Design review of the part built by this model. Coordinates are the model's own, in mm. A direction names the side the tool comes from. Coordinates: 2 decimals unless noted, no trailing zeros. Write each loop counter-clockwise with the first axis right and the second up, starting at its lowest first coordinate (ties: lowest second). Pieces come first, ordered by that corner, then holes. Notation, with made-up numbers: (1, -29.5) -> (56, -29.5) arc R34 cw to (56, 9.5) -> close; hole circle Ø5 at (41.5, 63.25). An arc over 180 degrees is marked (long way). Write item = value, one per line. Start each with the question number.
```python
from build123d import *

# Parameters (mm, degrees)
ESBO_O1_R                = 12.5
ESBO_O1_R_2              = 1.5
ESBO_O1_R_3              = 2.5
RESSALTO_EXTRUS_O2_DEPTH = 6
FILETE1_R                = 10
ESBO_O2_R                = 1.5
ESBO_O2_R_2              = 3
ESBO_O2_R_3              = 3.05
CORTE_EXTRUS_O1_DEPTH    = 238.194013415
ESBO_O3_R                = 3
CORTE_EXTRUS_O2_DEPTH    = 238.194013415


with BuildPart() as part:
    # Esboço1 → Ressalto-extrusão2 (new body)
    with BuildSketch(Plane.XY):
        Polygon((0, 0), (0, 215), (50, 215), (100, 0), align=None)
        with Locations((25, 195)):
            Circle(ESBO_O1_R, mode=Mode.SUBTRACT)
        with Locations((25, 211)):
            Circle(ESBO_O1_R_2, mode=Mode.SUBTRACT)
        with Locations((38.856406461, 203)):
            Circle(ESBO_O1_R_2, mode=Mode.SUBTRACT)
        with Locations((38.856406461, 187)):
            Circle(ESBO_O1_R_2, mode=Mode.SUBTRACT)
        with Locations((25, 179)):
            Circle(ESBO_O1_R_2, mode=Mode.SUBTRACT)
        with Locations((11.143593539, 187)):
            Circle(ESBO_O1_R_2, mode=Mode.SUBTRACT)
        with Locations((11.143593539, 203)):
            Circle(ESBO_O1_R_2, mode=Mode.SUBTRACT)
        with Locations((10, 45)):
            Circle(ESBO_O1_R_3, mode=Mode.SUBTRACT)
        with BuildLine():
            Line((20, 95), (20, 66))
            ThreePointArc((20, 66), (20.878679656, 63.878679656), (23, 63))
            Line((23, 63), (61.03739436, 63))
            ThreePointArc((61.03739436, 63), (63.386715693, 64.134339454), (63.959418441, 66.679540484))
            Line((63.959418441, 66.679540484), (57.215232395, 95.679540484))
            ThreePointArc((57.215232395, 95.679540484), (56.15886886, 97.349321333), (54.293208314, 98))
            Line((54.293208314, 98), (23, 98))
            ThreePointArc((23, 98), (20.878679656, 97.121320344), (20, 95))
        make_face(mode=Mode.SUBTRACT)
        with BuildLine():
            Line((20, 40), (20, 23))
            ThreePointArc((20, 23), (20.878679656, 20.878679656), (23, 20))
            Line((23, 20), (71.03739436, 20))
            ThreePointArc((71.03739436, 20), (73.386715693, 21.134339454), (73.959418441, 23.679540484))
            Line((73.959418441, 23.679540484), (70.005930069, 40.679540484))
            ThreePointArc((70.005930069, 40.679540484), (68.949566534, 42.349321333), (67.083905988, 43))
            Line((67.083905988, 43), (23, 43))
            ThreePointArc((23, 43), (20.878679656, 42.121320344), (20, 40))
        make_face(mode=Mode.SUBTRACT)
    extrude(amount=RESSALTO_EXTRUS_O2_DEPTH)

    # Filete1
    filete1_edges = [part.edges().sort_by_distance(p)[0] for p in [
        (0, 215, 3),
        (50, 215, 3),
    ]]
    fillet(filete1_edges, radius=FILETE1_R)

    # Esboço2 → Corte-extrusão1 (cut, through all)
    with BuildSketch(Plane.XY.offset(6)):
        with Locations((9.5, 137)):
            Circle(ESBO_O2_R)
        with Locations((90.5, 14.5)):
            Circle(ESBO_O2_R_2)
        with Locations((9.5, 112)):
            Circle(ESBO_O2_R)
        with Locations((9.5, 152)):
            Circle(ESBO_O2_R_3)
        with BuildLine():
            Line((13.5, 161.71), (13.5, 166.71))
            ThreePointArc((13.5, 166.71), (15, 168.21), (16.5, 166.71))
            Line((16.5, 166.71), (16.5, 161.71))
            ThreePointArc((16.5, 161.71), (15, 160.21), (13.5, 161.71))
        make_face()
        with BuildLine():
            Line((33.5, 161.71), (33.5, 166.71))
            ThreePointArc((33.5, 166.71), (35, 168.21), (36.5, 166.71))
            Line((36.5, 166.71), (36.5, 161.71))
            ThreePointArc((36.5, 161.71), (35, 160.21), (33.5, 161.71))
        make_face()
    extrude(amount=-CORTE_EXTRUS_O1_DEPTH, mode=Mode.SUBTRACT)

    # Esboço3 → Corte-extrusão2 (cut, through all)
    with BuildSketch(Plane.XY.offset(6)):
        with Locations((70.759810426, 80.398555206)):
            Circle(ESBO_O3_R)
    extrude(amount=-CORTE_EXTRUS_O2_DEPTH, mode=Mode.SUBTRACT)


solid = part.part
```
(1) Take a section at D-D, the plane z = 2.45. Count the separate pieces of the cut face and the enclosed holes in it, then the cut area to 3 significant figures.
(2) Take a section at B-B, the plane y = 91.5. State the section outline as (x, z) points.
(3) For pin 1 Ø22.5 at (x, y) = (25, 195) entering from +Z; pin 2 Ø1.5 at (y, z) = (164.5, 4.5) entering from +X, all flat-tipped, find the tip position at first contact; note any pin that passes through.
(4) Take a section at A-A, the plane x = 90.5. State the section outline as (y, z) points.
(5) Take a section at C-C, the plane x = 76.5. State the section outline as (y, z) points, then the cut area to 3 significant figures.
(6) For faces 4 (the face through (72, 32.1, 3)), 5 (the face through (2.85, 211.99, 3.04)), list the 3-axis set-ups (+Z, -Z, +X, -X, +Y, -Y) from which the entire face can be reached by the end or side of a thin tool; tool diameter is ignored.
(7) Mouldability with a two-part tool opening along X and no side actions: class faces 1 (the face through (9.46, 42.56, 2.96)), 2 (the face through (48.2, 212.89, 3.04)), 3 (the face through (26, 215, 3)) as pulls with the +X half, pulls with the -X half, needs draft (parallel to the pull), parting line crosses it, or undercut.
(8) For line 1 (Y direction, x = 25, z = 4.1); line 2 (X direction, y = 112, z = 4.75); line 3 (Y direction, x = 21.5, z = 4), list the stretches that pass through material, from the lowest coordinate up.
Report:
q1.separate_pieces = 1
q1.enclosed_holes = 17
q1.area = 12,800 mm2
q2.outline = (0, 0) -> (20, 0) -> (20, 6) -> (0, 6) -> close; (58.19, 0) -> (78.72, 0) -> (78.72, 6) -> (58.19, 6) -> close
q3.pin_1 = through
q3.pin_2 = 61.92
q4.outline = (0, 0) -> (11.5, 0) -> (11.5, 6) -> (0, 6) -> close; (17.5, 0) -> (40.85, 0) -> (40.85, 6) -> (17.5, 6) -> close
q5.outline = (0, 0) -> (101.05, 0) -> (101.05, 6) -> (0, 6) -> close
q5.area = 606 mm2
q6.face_4 = +Z, -Z
q6.face_5 = +Z, -Z, -X, +Y
q7.face_1 = undercut
q7.face_2 = pulls with the +X half
q7.face_3 = needs draft
q8.line_1 = 0 to 20, 43 to 63, 98 to 177.5, 180.5 to 182.5, 207.5 to 209.5, 212.5 to 215
q8.line_2 = 0 to 8, 11 to 73.95
q8.line_3 = 0 to 20.4, 42.6 to 63.4, 97.6 to 183, 207 to 215
